Autodesk Inventor part; units mm, degrees
ref_plane "YZ Plane" through (0, 0, 0) normal (1, 0, 0) x (0, 1, 0)
ref_plane "XZ Plane" through (0, 0, 0) normal (0, 1, 0) x (-1, 0, 0)
ref_plane "XY Plane" through (0, 0, 0) normal (0, 0, 1) x (1, 0, 0)
sketch "Sketch1" plane through (0, 0, 0) normal (0, 1, 0) x (-1, 0, 0)
  line L0 (0, 0) -> (-13.77, 0)
  line L1 (-13.77, 0) -> (-13.77, 6.9)
  line L2 (-13.77, 6.9) -> (0, 6.9)
  line L3 (0, 6.9) -> (0, 0)
  line L4 (3, -3) -> (-16.77, -3)
  line L5 (-16.77, -3) -> (-16.77, 9.9)
  line L6 (-16.77, 9.9) -> (3, 9.9)
  line L7 (3, 9.9) -> (3, -3)
  point P0 (-6.885, -3)
  point P1 (-6.885, 0)
  point P2 (3, 3.45)
  dimension "d0" = 13.77
  dimension "d1" = 6.9
  dimension "d2" = 3
  dimension "d3" = 3
  dimension "d4" = 3
  dimension "d5" = 3
extrude "Extrusion1" add sketch "Sketch1" along normal blind 8.8
sketch "Sketch2" plane through (0, 0, 0) normal (0, -1, 0) x (1, 0, 0)
  line L0 (-3, 9.9) -> (16.77, 9.9)
  line L1 (16.77, -3) -> (-3, -3)
  line L2 (-3, 9.9) -> (16.77, 9.9)
  line L3 (16.77, 9.9) -> (16.77, -3)
  line L4 (16.77, -3) -> (-3, -3)
  line L5 (-3, -3) -> (-3, 9.9)
  point P0 (0, 0)
  point P1 (16.77, 9.9)
extrude "Extrusion2" add sketch "Sketch2" along normal blind 3
sketch "Sketch3" plane through (0, 0, 0) normal (0, 1, 0) x (1, 0, 0)
  line L0 (0, -6.9) -> (0, 0)
  line L1 (13.77, -6.9) -> (0, -6.9)
  line L2 (0, 0) -> (8.3, 0)
  line L3 (8.3, 0) -> (8.3, -6.9)
  line L4 (8.3, -6.9) -> (0, -6.9)
  line L5 (0, -6.9) -> (0, 0)
  dimension "d10" = 8.3
extrude "Extrusion3" cut sketch "Sketch3" against normal blind 3
equation "\"d3\" = d2"
equation "\"d5\" = d4"
properties part number "switch test v02"
For this review, take the finished solid that the model builds, in its own axes (mm). A direction names the side the tool comes from. Coordinates: 2 decimals unless noted, no trailing zeros. Write each loop counter-clockwise with the first axis right and the second up, starting at its lowest first coordinate (ties: lowest second). Pieces come first, ordered by that corner, then holes.
(1) Tool access review of faces 1 (the face through (0, 3, 3)), 2 (the face through (9, -3, 4)), 3 (the face through (7, 3, 0)): name each direction out of +Z, -Z, +X, -X, +Y, -Y from which nothing blocks a thin tool from reaching the whole face with its end or side.
(2) Add section B-B on x = 0.5. Give the boundary of the cut face in (y, z), then the cut area to 3 significant figures.
(3) Add section A-A on z = 4. Give the boundary of the cut face in (x, y), then the cut area to 3 significant figures.
(4) Wall thickness on probe 1 along X at (y, z) = (3.75, 1); probe 2 along Z at (x, y) = (6.25, 4); probe 3 along X at (y, z) = (-2.5, 1): over which ranges is each line inside the solid? List them lowest first.
(5) Add section D-D on x = 8.75. Give the boundary of the cut face in (y, z), then the cut area to 3 significant figures.
(6) For pin 1 Ø1.6 at (x, z) = (9.5, 3.5) entering from +Y, flat-tipped, find the tip position at first contact; note if it passes through.
(7) Add section C-C on y = 4. Give the boundary of the cut face in (x, z).
(8) The part is to be moulded in two halves that separate along Z. For faces 4 (the face through (-3, 3, 4)), 5 (the face through (7, 3, 6.9)), 6 (the face through (7, 3, -3)), 7 (the face through (8.3, -1, 3)), say which applies: +Z half, -Z half, draft (parallel to the pull), parting line (faces both ways), or undercut.
Answer sheet:
1. face 1: +Y, -Y
1. face 2: +Z, -Z, +X, -X, -Y
1. face 3: +Y
2. outline: (-3, -3) - (8.8, -3) - (8.8, 0) - (-3, 0) - close; (-3, 6.9) - (8.8, 6.9) - (8.8, 9.9) - (-3, 9.9) - close
2. area: 70.8 mm2
3. outline: (-3, -3) - (0, -3) - (0, 8.8) - (-3, 8.8) - close; (8.3, -3) - (16.77, -3) - (16.77, 8.8) - (13.77, 8.8) - (13.77, 0) - (8.3, 0) - close
3. area: 87.2 mm2
4. probe 1: x = -3 to 0, 13.77 to 16.77
4. probe 2: z = -3 to 0, 6.9 to 9.9
4. probe 3: x = -3 to 0, 8.3 to 16.77
5. outline: (-3, -3) - (8.8, -3) - (8.8, 0) - (0, 0) - (0, 6.9) - (8.8, 6.9) - (8.8, 9.9) - (-3, 9.9) - close
5. area: 91.5 mm2
6. pin 1: stops at y = 0
7. outline: (-3, -3) - (16.77, -3) - (16.77, 9.9) - (-3, 9.9) - close; hole (0, 0) - (13.77, 0) - (13.77, 6.9) - (0, 6.9) - close
8. face 4: draft
8. face 5: undercut
8. face 6: -Z half
8. face 7: undercut
